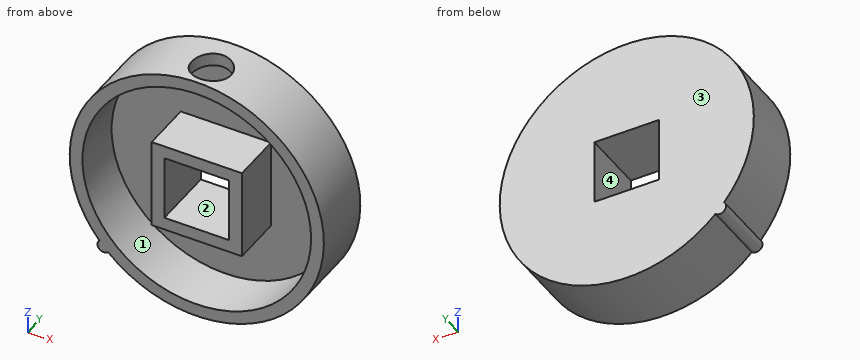
from build123d import *

# Parameters (mm, degrees)
SKETCH1_R           = 20
BOSS_EXTRUDE1_DEPTH = 10
SKETCH2_W           = 10.2
SKETCH2_H           = 10.2
CUT_EXTRUDE2_DEPTH  = 11
SHELL3_T            = -2
SKETCH3_R           = 3.1
CUT_EXTRUDE3_DEPTH  = 13.9
BOSS_EXTRUDE2_DEPTH = 10


with BuildPart() as part:
    # Sketch1 → Boss-Extrude1 (new body)
    with BuildSketch(Plane(origin=(0, 0, 0), x_dir=(1, 0, 0), z_dir=(0, 1, 0))):
        Circle(SKETCH1_R)
    extrude(amount=BOSS_EXTRUDE1_DEPTH)

    # Sketch2 → Cut-Extrude2 (cut, through all)
    with BuildSketch(Plane.XZ):
        Rectangle(SKETCH2_W, SKETCH2_H)
    extrude(amount=-CUT_EXTRUDE2_DEPTH, mode=Mode.SUBTRACT)

    # Shell3
    shell3_openings = [part.faces().sort_by_distance(p)[0] for p in [
        (0, 0, 0),
    ]]
    offset(amount=SHELL3_T, openings=shell3_openings, kind=Kind.INTERSECTION)

    # Sketch3 → Cut-Extrude3 (cut, through all)
    with BuildSketch(Plane.XY.offset(7.1)):
        with Locations((0, 4)):
            Circle(SKETCH3_R)
    extrude(amount=CUT_EXTRUDE3_DEPTH, mode=Mode.SUBTRACT)

    # Sketch4 → Boss-Extrude2 (add)
    with BuildSketch(Plane(origin=(0, 10, 0), x_dir=(1, 0, 0), z_dir=(0, 1, 0))):
        with BuildLine():
            Line((-13.960317173, 14.321646009), (-15.320888862, 12.855752194))
            ThreePointArc((-15.320888862, 12.855752194), (-15.373549926, 14.268984946), (-13.960317173, 14.321646009))
        make_face()
    extrude(amount=-BOSS_EXTRUDE2_DEPTH)


solid = part.part
Can you work these out from the model? Positions are in its coordinate system, mm. Face numbers are marked on the shaded views. A direction names the side the tool comes from. Round coordinates to 2 decimals unless told otherwise and drop trailing zeros. Loops run counter-clockwise (first coordinate to the right, second up) from the corner with the lowest first, then second, coordinate; pieces in that order, holes last. Notation, with made-up numbers: (-14.75, 8) - (23.25, 8) arc R29 cw to (23.25, 41) - close; hole circle Ø5 at (89.25, 19.25). An arc over 180 degrees is marked (long way). Answer in a Markdown table with one row per item. Add a question column.
Q1. Which directions (+Z, -Z, +X, -X, +Y, -Y) give clear straight access to the entire face, cutting with the end or side of a thin tool? Please do the marked faces 1 and 2.
Q2. We'd pull the mould along X, two halves only. Please class the marked faces 3 and 4: pulls with the +X half, pulls with the -X half, needs draft (parallel to the pull), parting line crosses it, or undercut.
Q3. I want a section at C-C on z = 0. List the corners of the cut face in (x, y) for me.
Q4. I want a section at D-D on x = 16. List the corners of the cut face in (y, z) for me, and give its area (3 significant figures).
Q5. I want a section at B-B on y = 6.5. List the corners of the cut face in (x, z) for me.
Q6. I need wall thicknesses on L1, parallel to Z at x = 2.5, y = 0.75; L2, parallel to Z at x = 0, y = 3.75; L3, parallel to Z at x = -4, y = 4.75. Which ranges of each line are inside material? Lowest first, please.
Q7. I want a section at A-A on x = 0. List the corners of the cut face in (y, z) for me, and give its area (3 significant figures).
Q8. For pin 1 Ø6 at (y, z) = (2.5, -6.5) entering from +X; pin 2 Ø3 at (x, y) = (-1.5, 4.5) entering from -Z; pin 3 Ø2.5 at (y, z) = (3, 3.5) entering from +X; pin 4 Ø2.5 at (x, y) = (1, 2.5) entering from +Z, each with a flat end and sliding along its axis, tell me the tip position at first contact or that it passes through.
A:
| question | item | result |
|---|---|---|
| 1 | face 1 | -Y |
| 1 | face 2 | +Y, -Y |
| 2 | face 3 | needs draft |
| 2 | face 4 | undercut |
| 3 | outline | (-20, 0) - (-18, 0) - (-18, 8) - (-7.1, 8) - (-7.1, 0) - (-5.1, 0) - (-5.1, 10) - (-20, 10) - close; (5.1, 0) - (7.1, 0) - (7.1, 8) - (18, 8) - (18, 0) - (20, 0) - (20, 10) - (5.1, 10) - close |
| 4 | outline | (0, -12) - (10, -12) - (10, 12) - (0, 12) - (0, 8.25) - (8, 8.25) - (8, -8.25) - (0, -8.25) - close |
| 4 | area | 108 mm^2 |
| 5 | outline | (-15.32, -12.86) arc R1 ccw to (-13.96, -14.32) arc R20 ccw (long way) to (1.83, 19.92) - (1.83, 17.91) arc R18 cw (long way) to (-1.83, 17.91) - (-1.83, 19.92) arc R20 ccw to start; (-7.1, -7.1) - (7.1, -7.1) - (7.1, 7.1) - (-7.1, 7.1) - close; hole (-5.1, -5.1) - (5.1, -5.1) - (5.1, 5.1) - (-5.1, 5.1) - close |
| 6 | L1 | -19.84 to -17.83, -7.1 to -5.1, 5.1 to 7.1, 17.83 to 19.84 |
| 6 | L2 | -20 to -18, -7.1 to -5.1, 5.1 to 7.1 |
| 6 | L3 | -19.6 to -17.55, -7.1 to -5.1, 5.1 to 7.1, 17.55 to 19.6 |
| 7 | outline | (0, -20) - (10, -20) - (10, -5.1) - (0, -5.1) - (0, -7.1) - (8, -7.1) - (8, -18) - (0, -18) - close; (0, 5.1) - (10, 5.1) - (10, 20) - (7.1, 20) - (7.1, 18) - (8, 18) - (8, 7.1) - (0, 7.1) - close; (0, 18) - (0.9, 18) - (0.9, 20) - (0, 20) - close |
| 7 | area | 111 mm^2 |
| 8 | pin 1 | x = 19.69 |
| 8 | pin 2 | z = -20 |
| 8 | pin 3 | x = 19.87 |
| 8 | pin 4 | z = 7.1 |
